Study the drawing (mm; zero at the part's minimum x, y, z) and answer. Coordinates: 2 decimals unless noted, no trailing zeros. Order: outer loops, then holes, each group sorted by start corner. A loop starts at its lowest first (then second) coordinate and runs counter-clockwise, first axis right, second up. Notation, with made-up numbers: M 12.25,59 L 61.25,59 A24 cw 61.25,80 Z; hole C 27,5 d6. An arc over 180 degrees is marked long. One line per item, written item: value. Start each with the question number.
Q1. Each of these flat-tipped pins is pushed along its axis until it touches: pin 1 Ø1.5 at (y, z) = (17, 73.5) entering from -X; pin 2 Ø4 at (y, z) = (18.5, 75) entering from +X; pin 3 Ø2.5 at (x, z) = (64, 73.5) entering from -Y. Where does it stop, or does it pass through?
Q2. The part is cut by section B-B on x = 73. Give the vertices of the cut face in (y, z), then the cut area to 3 significant figures.
Q3. The part is cut by section A-A on y = 11.5. Give the vertices of the cut face in (x, z).
Q4. A straight line is drawn through the part: line 1 along Z through (x, y) = (70.5, 27). Find the intervals that lie inside material, in ascending order. Write a range as [from, to].
Q5. Determine the mould class of the marked faces 1, 2 and 3 for opening direction Y: pulls with the +Y half, pulls with the -Y half, needs draft (parallel to the pull), parting line crosses it, or undercut.
Q6. The part is cut by section D-D on y = 26.75. Give the vertices of the cut face in (x, z).
Q7. The part is cut by section C-C on x = 6. Give the vertices of the cut face in (y, z), then the cut area to 3 significant figures.
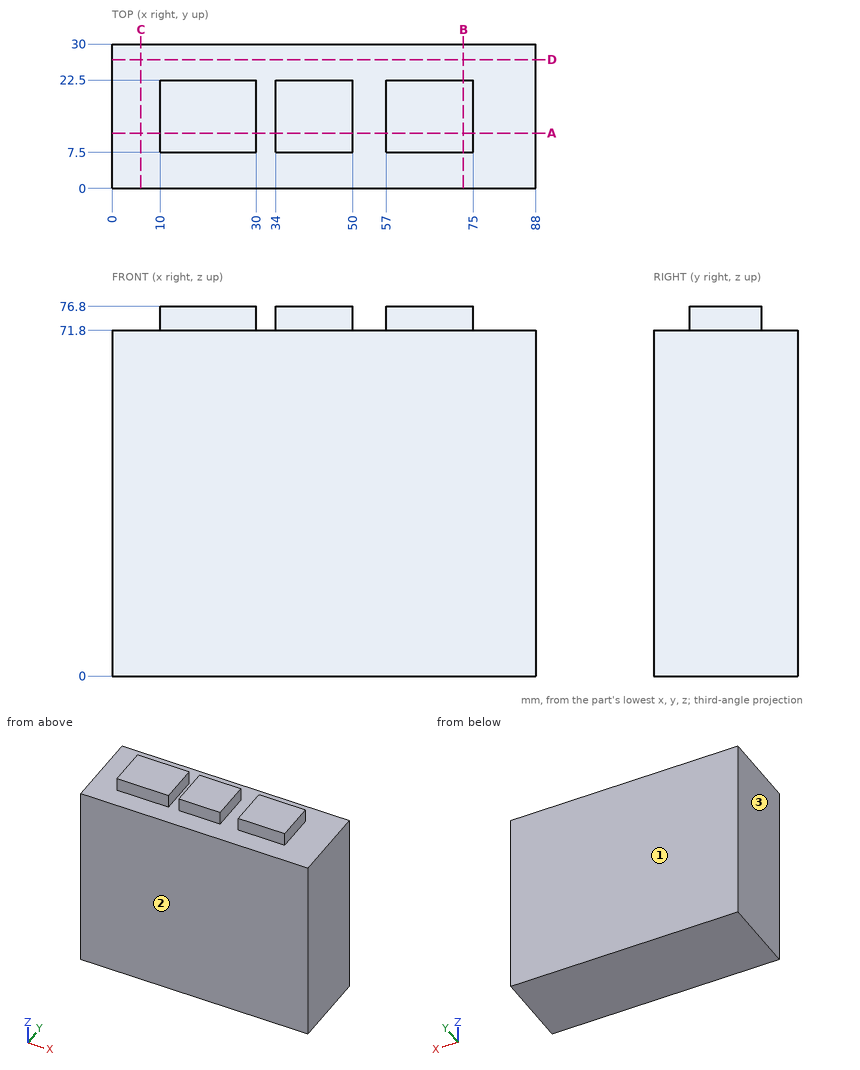
Output:
1. pin 1: stops at x = 10
1. pin 2: stops at x = 75
1. pin 3: stops at y = 7.5
2. outline: M 0,0 L 30,0 L 30,71.8 L 22.5,71.8 L 22.5,76.8 L 7.5,76.8 L 7.5,71.8 L 0,71.8 Z
2. area: 2,230 mm^2
3. outline: M 0,0 L 88,0 L 88,71.8 L 75,71.8 L 75,76.8 L 57,76.8 L 57,71.8 L 50,71.8 L 50,76.8 L 34,76.8 L 34,71.8 L 30,71.8 L 30,76.8 L 10,76.8 L 10,71.8 L 0,71.8 Z
4. line 1: z = [0, 71.8]
5. face 1: pulls with the +Y half
5. face 2: pulls with the -Y half
5. face 3: needs draft
6. outline: M 0,0 L 88,0 L 88,71.8 L 0,71.8 Z
7. outline: M 0,0 L 30,0 L 30,71.8 L 0,71.8 Z
7. area: 2,150 mm^2
